```python
from build123d import *

# Parameters (mm, degrees)
BOSS_EXTRUDE1_DEPTH  = 1.778
M3_CLEARANCE_HOLE1_D = 3.2
SKETCH4_W            = 2.54
SKETCH4_H            = 9.144
BOSS_EXTRUDE2_DEPTH  = 1.143
CUT_EXTRUDE1_DEPTH   = 0.508


with BuildPart() as part:
    # Sketch1 → Boss-Extrude1 (new body)
    with BuildSketch(Plane(origin=(0, 0, 0), x_dir=(1, 0, 0), z_dir=(0, 1, 0))):
        Polygon((0, 15.367), (0, 0), (8.255, 0), (8.255, -3.81), (14.605, -3.81), (14.605, 0), (22.86, 0), (22.86, 15.367), (19.685, 15.367), (19.685, 16.637), (1.143, 16.637), (1.143, 15.367), align=None)
    extrude(amount=BOSS_EXTRUDE1_DEPTH)

    # M3 Clearance Hole1 (through all)
    with Locations(Plane(origin=(0, 1.778, 0), x_dir=(1, 0, 0), z_dir=(0, 1, 0))):
        with Locations((11.43, -0.888075369)):
            Hole(M3_CLEARANCE_HOLE1_D / 2)

    # Sketch4 → Boss-Extrude2 (add)
    with BuildSketch(Plane.XZ):
        with Locations((16.51, -8.874849992)):
            Rectangle(SKETCH4_W, SKETCH4_H)
        with Locations((1.27, -8.874849992)):
            Rectangle(SKETCH4_W, SKETCH4_H)
    extrude(amount=BOSS_EXTRUDE2_DEPTH)

    # Sketch6 → Cut-Extrude1 (cut)
    # profile 1 of 2: a face of its own
    with BuildSketch(Plane.XZ):
        Polygon((7.792887548, -6.937433067), (7.970271363, -6.937433067), (7.970271363, -9.315638195), (8.374117516, -9.315638195), (8.374117516, -9.719484349), (7.970271363, -9.719484349), (7.970271363, -10.527176657), (7.521553414, -10.527176657), (7.521553414, -9.719484349), (5.906168798, -9.719484349), align=None)
        Polygon((7.521553414, -9.315638195), (7.521553414, -7.923911433), (6.630427613, -9.315638195), align=None, mode=Mode.SUBTRACT)
    # profile 2 of 2: a face of its own
    with BuildSketch(Plane.XZ):
        with BuildLine():
            Line((10.931809824, -7.027176657), (10.931809824, -7.431022811))
            Line((10.931809824, -7.431022811), (9.78197008, -7.431022811))
            Line((9.78197008, -7.431022811), (9.594069439, -8.260449894))
            add(Edge.make_bspline(
                [(9.594069439, -8.260449894), (9.615990404, -8.249885481), (9.661103923, -8.228143835), (9.736526874, -8.209200238), (9.818414717, -8.195871542), (9.875622645, -8.194537138), (9.905367516, -8.193843324)],
                knots=[0, 0, 0, 0, 0.906577793, 1.865744317, 2.890308309, 4, 4, 4, 4], degree=3))
            add(Edge.make_bspline(
                [(9.905367516, -8.193843324), (9.947495326, -8.194614643), (10.030206236, -8.196129001), (10.150750761, -8.213051384), (10.265618253, -8.23840338), (10.373863762, -8.27622385), (10.476723422, -8.322782641), (10.573081318, -8.381044204), (10.66283737, -8.450020231), (10.745871527, -8.528536241), (10.821549898, -8.614059011), (10.886547349, -8.706415291), (10.942889062, -8.802907042), (10.98754851, -8.905201736), (11.022834099, -9.012241242), (11.047928323, -9.124472926), (11.063881421, -9.241560513), (11.065569539, -9.321428782), (11.066425209, -9.361912234)],
                knots=[0, 0, 0, 0, 1.094894284, 2.149641875, 3.159658044, 4.149576056, 5.125966368, 6.091225838, 7.071072142, 8.064343292, 9.05924964, 10.03573454, 10.996966885, 11.96032995, 12.932910184, 13.923798045, 14.947619342, 16, 16, 16, 16], degree=3))
            add(Edge.make_bspline(
                [(11.066425209, -9.361912234), (11.06576722, -9.390201132), (11.064465608, -9.446161323), (11.057683043, -9.529370503), (11.044736374, -9.610784817), (11.027546624, -9.691033112), (11.003860501, -9.769427433), (10.97689686, -9.84701), (10.943769877, -9.922543999), (10.905950095, -9.995997939), (10.863989349, -10.066834257), (10.817788624, -10.134193652), (10.767242359, -10.197537594), (10.712171199, -10.256335904), (10.654080504, -10.312100821), (10.59145493, -10.363376929), (10.524472443, -10.410379599), (10.454088485, -10.453622636), (10.380336705, -10.492689435), (10.302783653, -10.525035952), (10.223354637, -10.554425694), (10.140085205, -10.576431812), (10.054545441, -10.594949081), (9.965708783, -10.607237727), (9.874197953, -10.615249641), (9.812135855, -10.616356991), (9.780567837, -10.616920247)],
                knots=[0, 0, 0, 0, 1.012275937, 2.002451767, 2.98397589, 3.959820946, 4.936095762, 5.911940818, 6.896771482, 7.884012822, 8.866284557, 9.840372785, 10.804070441, 11.762530572, 12.720625922, 13.68308951, 14.655094125, 15.646011038, 16.637104318, 17.63729087, 18.650257215, 19.66446511, 20.715636712, 21.77986274, 22.870722459, 24, 24, 24, 24], degree=3))
            add(Edge.make_bspline(
                [(9.780567837, -10.616920247), (9.74501295, -10.616066651), (9.67487051, -10.614382685), (9.571851951, -10.602438699), (9.473022547, -10.582173288), (9.378801083, -10.553163592), (9.288486547, -10.516777369), (9.202848927, -10.471765507), (9.121555434, -10.418531983), (9.044501382, -10.358091639), (8.974225046, -10.289145312), (8.909445749, -10.214922365), (8.854253251, -10.132690105), (8.805700589, -10.044717841), (8.763983147, -9.950290059), (8.73079481, -9.849227723), (8.704256829, -9.74191356), (8.693649883, -9.66772079), (8.68822008, -9.62974076)],
                knots=[0, 0, 0, 0, 1.049569621, 2.070583864, 3.057046508, 4.023914414, 4.977170942, 5.927726879, 6.875021894, 7.842677272, 8.813672282, 9.777581439, 10.74592533, 11.731059957, 12.74126976, 13.788569057, 14.867946107, 16, 16, 16, 16], degree=3))
            Line((8.68822008, -9.62974076), (9.126421202, -9.62974076))
            add(Edge.make_bspline(
                [(9.126421202, -9.62974076), (9.134761141, -9.66642032), (9.150417161, -9.735276452), (9.184050813, -9.829097607), (9.220098703, -9.908893266), (9.264188523, -9.974152261), (9.314792456, -10.027719829), (9.370959214, -10.074218016), (9.432665368, -10.115927928), (9.500597498, -10.150550709), (9.572171535, -10.17860074), (9.646539379, -10.198177788), (9.722199143, -10.210487725), (9.773277222, -10.212212404), (9.798797004, -10.213074093)],
                knots=[0, 0, 0, 0, 1.385459112, 2.600831482, 3.66841355, 4.605180919, 5.48910649, 6.376050311, 7.288896949, 8.229144678, 9.181161654, 10.117453426, 11.059436513, 12, 12, 12, 12], degree=3))
            add(Edge.make_bspline(
                [(9.798797004, -10.213074093), (9.826403635, -10.212147278), (9.880907737, -10.210317457), (9.9612011, -10.199363174), (10.03799139, -10.179100678), (10.112387313, -10.152836823), (10.183089403, -10.117064359), (10.251833101, -10.075295418), (10.316111719, -10.02400433), (10.377721757, -9.966974677), (10.434150348, -9.903805344), (10.483285658, -9.835553671), (10.525200218, -9.763590176), (10.558602509, -9.687436209), (10.585711354, -9.607789577), (10.60434487, -9.524106273), (10.615970273, -9.436561106), (10.617120647, -9.376907087), (10.61770726, -9.346487554)],
                knots=[0, 0, 0, 0, 0.99750234, 1.969380735, 2.919490565, 3.862219911, 4.813679117, 5.776605688, 6.762898166, 7.778387729, 8.806918829, 9.816812977, 10.811632172, 11.809420289, 12.815921014, 13.846113939, 14.901663155, 16, 16, 16, 16], degree=3))
            add(Edge.make_bspline(
                [(10.61770726, -9.346487554), (10.61700976, -9.319346395), (10.615640161, -9.266052481), (10.605607573, -9.18816159), (10.589693867, -9.113863306), (10.566569889, -9.043856082), (10.536844883, -8.977752547), (10.500292329, -8.915975577), (10.457023625, -8.858181151), (10.408363657, -8.804181975), (10.353279511, -8.755933356), (10.294135331, -8.712751732), (10.2291352, -8.677827545), (10.160623288, -8.647941478), (10.087014842, -8.626099622), (10.009628455, -8.608500045), (9.927054225, -8.6000444), (9.870558601, -8.59848814), (9.841565433, -8.597689477)],
                knots=[0, 0, 0, 0, 1.071512717, 2.104004018, 3.095982969, 4.067795438, 5.009520676, 5.952827242, 6.895998369, 7.856350385, 8.817411605, 9.782937659, 10.74115891, 11.725120868, 12.729302161, 13.768330494, 14.854722481, 16, 16, 16, 16], degree=3))
            add(Edge.make_bspline(
                [(9.841565433, -8.597689477), (9.816772294, -8.598284479), (9.764721648, -8.599533624), (9.683271646, -8.608565862), (9.594637888, -8.622772307), (9.498960529, -8.6424206), (9.396147628, -8.66801835), (9.286074253, -8.699036547), (9.168618604, -8.735231112), (9.088481339, -8.762914245), (9.047194439, -8.777176657)],
                knots=[0, 0, 0, 0, 0.727614075, 1.527550888, 2.402655696, 3.361819828, 4.39328773, 5.511706796, 6.718025739, 8, 8, 8, 8], degree=3))
            Line((9.047194439, -8.777176657), (9.41458226, -7.027176657))
            Line((9.41458226, -7.027176657), (10.931809824, -7.027176657))
        make_face()
    extrude(amount=-CUT_EXTRUDE1_DEPTH, mode=Mode.SUBTRACT)


solid = part.part
```
Model file for the job. Use its own axes, mm. A direction names the side the tool comes from. Give positions to 0.01 mm unless a question says otherwise; leave off trailing zeros. Loops run counter-clockwise (first coordinate to the right, second up) from the corner with the lowest first, then second, coordinate; pieces in that order, holes last. Notation, with made-up numbers: (76, 4.5) -> (90, 4.5) arc R11 cw to (90, 12.5) -> close; hole circle Ø2 at (-2.5, 87). An arc over 180 degrees is marked (long way). Write each question's results on one line, items separated by ' | '.
(1) Cut at C-C on y = 0.8. List the corners of the cut face in (x, z) (3 decimals).
Geometry results:
outline: (0, -15.367) -> (1.143, -15.367) -> (1.143, -16.637) -> (19.685, -16.637) -> (19.685, -15.367) -> (22.86, -15.367) -> (22.86, 0) -> (14.605, 0) -> (14.605, 3.81) -> (8.255, 3.81) -> (8.255, 0) -> (0, 0) -> close; hole circle Ø3.2 at (11.43, 0.888)
(2) Cut at D-D on x = 18.25. List the corners of the cut face in (y, z).
Geometry results:
outline: (0, -16.64) -> (1.78, -16.64) -> (1.78, 0) -> (0, 0) -> close
(3) Pull direction X, two halves, no side cores. Call faces 1 (the flat face through (16.5, -0.6, -4.303)), 2 (the flat face through (19.685, 1, -16)), 3 (the flat face through (6.836, 0.25, -8.348)): released by +X, released by -X, zero draft, split by the parting line, or undercut.
Geometry results:
face 1: zero draft | face 2: released by +X | face 3: undercut
(4) Cut at B-B on z = 1.75. List the corners of the cut face in (x, y) (3 decimals), and give its area (3 significant figures).
Geometry results:
outline: (8.255, 0) -> (10.082, 0) -> (10.082, 1.778) -> (8.255, 1.778) -> close; (12.778, 0) -> (14.605, 0) -> (14.605, 1.778) -> (12.778, 1.778) -> close | area: 6.50 mm²
(5) Cut at A-A on x = 11.43. List the corners of the cut face in (y, z).
Geometry results:
outline: (0, -16.64) -> (1.78, -16.64) -> (1.78, -0.71) -> (0, -0.71) -> close; (0, 2.49) -> (1.78, 2.49) -> (1.78, 3.81) -> (0, 3.81) -> close
(6) Flat gauge pins, fed straight in: pin 1 Ø1.2 at (x, z) = (10, -9.5) entering from -Y; pin 2 Ø0.6 at (y, z) = (0.5, -16) entering from -X; pin 3 Ø0.9 at (x, y) = (16, -0.5) entering from +Z. Where does each tip first touch, or does it go through?
Geometry results:
pin 1: stops at y = 0 | pin 2: stops at x = 1.14 | pin 3: stops at z = -4.3
(7) Tool access for faces 4 (the flat face through (19, 1, 0)), 5 (the flat face through (7.08, 0.25, -8.61)), 6 (the flat face through (1.3, -0.6, -13.447)), 7 (the flat face through (8.255, 1, 2)): list every direction of +Z, -Z, +X, -X, +Y, -Y with a clear straight run to the whole face (end or side of a thin tool).
Geometry results:
face 4: +Z, +X, +Y, -Y | face 5: -Y | face 6: -Z, +X, -X, -Y | face 7: +Z, -X, +Y, -Y
(8) Probe line 1 along X through (y, z) = (-0.05, -6.25); line 2 along Y through (x, z) = (2, -1); line 3 along Z through (x, y) = (11.43, 1.4). List the from-to ranges inside material, lowest first.
Geometry results:
line 1: x = 0 to 2.54, 15.24 to 17.78 | line 2: y = 0 to 1.78 | line 3: z = -16.64 to -0.71, 2.49 to 3.81
